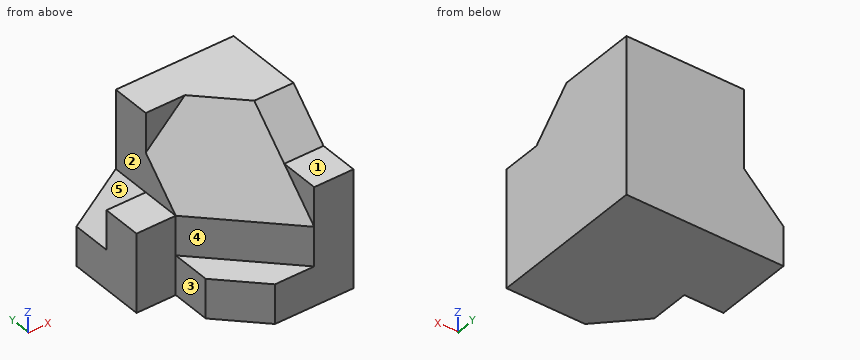
from build123d import *

# Parameters (mm, degrees)
SKETCH1_W            = 40
SKETCH1_H            = 40
BOSS_EXTRUDE1_DEPTH  = 20
BOSS_EXTRUDE3_DEPTH  = 10
SKETCH3_W            = 10
SKETCH3_H            = 30
BOSS_EXTRUDE5_DEPTH  = 10
BOSS_EXTRUDE6_DEPTH  = 10
SKETCH5_W            = 10
SKETCH5_H            = 40
CUT_EXTRUDE3_DEPTH   = 25
CUT_EXTRUDE4_DEPTH   = 25
CUT_EXTRUDE5_DEPTH   = 10
SKETCH9_W            = 20
SKETCH9_H            = 20
BOSS_EXTRUDE7_DEPTH  = 10
CUT_EXTRUDE6_DEPTH   = 10
BOSS_EXTRUDE8_DEPTH  = 10
SKETCH12_W           = 20
SKETCH12_H           = 10
BOSS_EXTRUDE9_DEPTH  = 20
BOSS_EXTRUDE10_DEPTH = 20
BOSS_EXTRUDE11_DEPTH = 20
BOSS_EXTRUDE12_DEPTH = 17


with BuildPart() as part:
    # Sketch1 → Boss-Extrude1 (new body)
    with BuildSketch(Plane.XY):
        with Locations((20, 20)):
            Rectangle(SKETCH1_W, SKETCH1_H)
    extrude(amount=BOSS_EXTRUDE1_DEPTH)

    # Sketch3 → Boss-Extrude5 (add)
    with BuildSketch(Plane(origin=(40, 0, 0), x_dir=(0, 0, -1), z_dir=(1, 0, 0))):
        with Locations((-25, 25)):
            Rectangle(SKETCH3_W, SKETCH3_H)
    extrude(amount=-BOSS_EXTRUDE5_DEPTH)



with BuildPart() as body_2:
    # Sketch2 → Boss-Extrude3 (new body)
    with BuildSketch(Plane(origin=(40, 0, 0), x_dir=(0, 0, -1), z_dir=(1, 0, 0))):
        Polygon((-30, 10), (-20, 0), (-30, 0), align=None)
    extrude(amount=-BOSS_EXTRUDE3_DEPTH)


with BuildPart() as part_1:
    add(part.part)

    add(body_2.part)  # Boss-Extrude6 merges body 2
    # Sketch4 → Boss-Extrude6 (add)
    with BuildSketch(Plane(origin=(40, 0, 0), x_dir=(0, 0, -1), z_dir=(1, 0, 0))):
        Polygon((-20, 0), (-20, 10), (-30, 10), align=None)
    extrude(amount=-BOSS_EXTRUDE6_DEPTH)

    # Sketch5 → Cut-Extrude3 (cut)
    with BuildSketch(Plane.XY.offset(20)):
        with Locations((5, 20)):
            Rectangle(SKETCH5_W, SKETCH5_H)
    extrude(amount=-CUT_EXTRUDE3_DEPTH, mode=Mode.SUBTRACT)

    # Sketch7 → Cut-Extrude4 (cut)
    with BuildSketch(Plane.XY.offset(20)):
        Polygon((10, 10), (20, 0), (10, 0), align=None)
    extrude(amount=-CUT_EXTRUDE4_DEPTH, mode=Mode.SUBTRACT)

    # Sketch8 → Cut-Extrude5 (cut)
    with BuildSketch(Plane.XY.offset(20)):
        Polygon((30, 0), (10, 20), (10, 10), (20, 0), align=None)
    extrude(amount=-CUT_EXTRUDE5_DEPTH, mode=Mode.SUBTRACT)

    # Sketch9 → Boss-Extrude7 (add)
    with BuildSketch(Plane.ZY.offset(-10)):
        with Locations((10, 30)):
            Rectangle(SKETCH9_W, SKETCH9_H)
    extrude(amount=BOSS_EXTRUDE7_DEPTH)

    # Sketch10 → Cut-Extrude6 (cut)
    with BuildSketch(Plane(origin=(0, 40, 0), x_dir=(1, 0, 0), z_dir=(0, 1, 0))):
        Polygon((10, -20), (0, -10), (0, -20), align=None)
    extrude(amount=-CUT_EXTRUDE6_DEPTH, mode=Mode.SUBTRACT)

    # Sketch11 → Boss-Extrude8 (add)
    with BuildSketch(Plane.ZY.offset(-30)):
        Polygon((30, 10), (40, 20), (40, 40), (30, 40), align=None)
    extrude(amount=-BOSS_EXTRUDE8_DEPTH)

    # Sketch12 → Boss-Extrude9 (add)
    with BuildSketch(Plane.ZY.offset(-30)):
        with Locations((30, 35)):
            Rectangle(SKETCH12_W, SKETCH12_H)
    extrude(amount=BOSS_EXTRUDE9_DEPTH)

    # Sketch13 → Boss-Extrude10 (add)
    with BuildSketch(Plane.XY.offset(40)):
        Polygon((30, 20), (20, 30), (30, 30), align=None)
    extrude(amount=-BOSS_EXTRUDE10_DEPTH)

    # Sketch16 → Boss-Extrude11 (add)
    with BuildSketch(Plane.ZY.offset(-10)):
        Polygon((20, 20), (30, 30), (20, 30), align=None)
    extrude(amount=-BOSS_EXTRUDE11_DEPTH)

    # Sketch17 → Boss-Extrude12 (add)
    with BuildSketch(Plane(origin=(3.333333333, 3.333333333, -3.333333333), x_dir=(-0.816496581, 0.40824829, -0.40824829), z_dir=(0.577350269, 0.577350269, -0.577350269))):
        Polygon((-32.659863237, 42.426406871), (-20.412414523, 49.497474683), (-8.164965809, 42.426406871), (-8.164965809, 28.284271247), (-32.659863237, 14.142135624), align=None)
    extrude(amount=BOSS_EXTRUDE12_DEPTH)


solid = part_1.part
Can you work these out from the model? Positions are in its coordinate system, mm. Face numbers are marked on the shaded views. A direction names the side the tool comes from. Give positions to 0.01 mm unless a question says otherwise; leave off trailing zeros. Order: outer loops, then holes, each group sorted by start corner. A loop starts at its lowest first (then second) coordinate and runs counter-clockwise, first axis right, second up. Notation, with made-up numbers: (-1, 68.5) - (7, 68.5) arc R17 cw to (7, 82.5) - close; hole circle Ø2 at (-6.75, 61.5). An arc over 180 degrees is marked (long way). Write each question's results on one line, items separated by ' | '.
1) I'm going to push flat-ended pins straight in: pin 1 Ø6 at (y, z) = (28.5, 25.5) entering from -X; pin 2 Ø5 at (x, z) = (3, 10.5) entering from -Y; pin 3 Ø1.5 at (x, z) = (20, 27) entering from -Y; pin 4 Ø1 at (x, y) = (12, 5.5) entering from +Z. Where does each tip first touch, or does it pass through?
Final values:
pin 1: stops at x = 10 | pin 2: stops at y = 20 | pin 3: stops at y = 15.94 | pin 4: passes through
2) Suppose I cut it at A-A, the plane z = 17. Write out the boundary of the cut face in (x, y), then the cut area to 3 significant figures.
Final values:
outline: (0, 20) - (10, 20) - (30, 0) - (40, 0) - (40, 40) - (7, 40) - (7, 30) - (0, 30) - close | area: 1,130 mm^2
3) Suppose I cut it at D-D, the plane z = 8. Write out the boundary of the cut face in (x, y).
Final values:
outline: (0, 20) - (10, 20) - (10, 10) - (20, 0) - (40, 0) - (40, 40) - (0, 40) - close
4) Please list where these lines run through material, in increasing order: line 1 along Y through (x, z) = (14, 37.5); line 2 along X through (y, z) = (37.5, 24.5). Write a range as [from, to].
Final values:
line 1: y = [30, 40] | line 2: x = [10, 40]
5) On a 3-axis mill with a long thin cutter (end or side, diameter ignored), from which of +Z, -Z, +X, -X, +Y, -Y can I reach the whole of each face in a straight line? I mean the marked faces 1, 2, 3, 4 and 5. Say none if no direction works.
Final values:
face 1: +Z, +X, -X, -Y | face 2: +Z, -X, +Y, -Y | face 3: +Z, -Z, -X, -Y | face 4: +Z, -X, -Y | face 5: +Z, -X, +Y
6) Suppose I cut it at B-B, the plane x = 27. Write out the boundary of the cut face in (y, z), then the cut area to 3 significant figures.
Final values:
outline: (0, 0) - (40, 0) - (40, 40) - (23, 40) - (3, 20) - (3, 10) - (0, 10) - close | area: 1,310 mm^2
7) Suppose I cut it at C-C, the plane y = 8.5. Write out the boundary of the cut face in (x, z), then the cut area to 3 significant figures.
Final values:
outline: (11.5, 0) - (40, 0) - (40, 30) - (30, 30) - (30, 28.5) - (21.5, 20) - (21.5, 10) - (11.5, 10) - close | area: 606 mm^2
